For this review, take the finished solid that the model builds, in its own axes (mm). Face numbers are marked on the shaded views. A direction names the side the tool comes from. Round coordinates to 2 decimals unless told otherwise and drop trailing zeros. Write each loop counter-clockwise with the first axis right and the second up, starting at its lowest first coordinate (ties: lowest second). Pieces come first, ordered by that corner, then holes. Notation, with made-up numbers: (23, -32) -> (40, -32) arc R15 cw to (40, -13) -> close; hole circle Ø4 at (-10.5, -26). An arc over 180 degrees is marked (long way). Answer as CSV lines item,"result". Start each with the question number.
Item 1: Machinability: for the marked faces 5, 6, 7, 8 and 9, which of the approach directions +Z, -Z, +X, -X, +Y, -Y give a long, thin tool a straight path to every point of the face, cutting with its end or side? Answer none if there is none.
Item 2: For pin 1 Ø4 at (y, z) = (-1.5, -1.5) entering from +X; pin 2 Ø5 at (x, z) = (15, 1) entering from -Y; pin 3 Ø3 at (y, z) = (-8, -0.5) entering from -X, all flat-tipped, find the tip position at first contact; note any pin that passes through.
Item 3: Take a section at C-C on y = -9. Give the boundary of the cut face in (x, z).
Item 4: Take a section at D-D on x = 5. Give the boundary of the cut face in (y, z).
Item 5: Wall thickness on probe 1 along X at (y, z) = (-2.5, -2.25); probe 2 along X at (y, z) = (-2.5, -5.65); probe 3 along Z at (x, y) = (40, -11.5): over which ranges is each line inside the solid? List them lowest first. Write a range as from..to.
Item 6: Take a section at B-B on z = -0.5. Give the boundary of the cut face in (x, y).
Item 7: Mouldability with a two-part tool opening along Z and no side actions: class the marked faces 1, 2, 3 and 4 as +Z half, -Z half, draft (parallel to the pull), parting line (faces both ways), or undercut.
Item 8: Take a section at A-A on x = 34. Give the boundary of the cut face in (y, z), then the cut area to 3 significant figures.
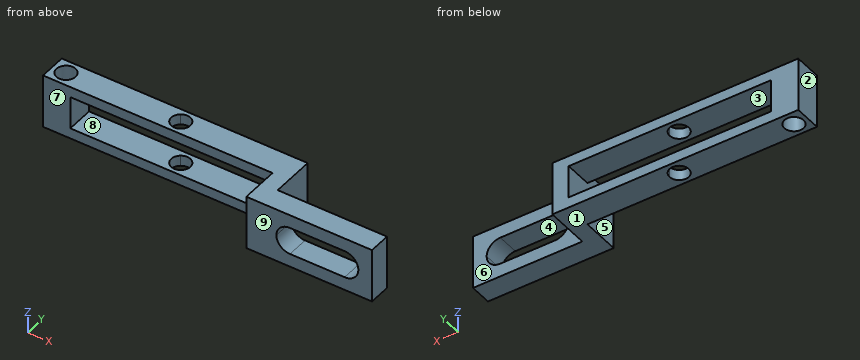
```python
from build123d import *

# Parameters (mm, degrees)
F0_W     = 3
F0_H     = 3
F1_DEPTH = 5
F3_DEPTH = 25
F4_W     = 3
F4_H     = 9.87
F5_DEPTH = 7
F6_W     = 4
F6_H     = 9.87
F7_DEPTH = 20
F9_DEPTH = 25


with BuildPart() as f1:
    # F0 (on Front) → F1 (new body)
    with BuildSketch(Plane.XZ):
        Polygon((-18.4640498906, -4.8765387449), (-18.4640498906, -6.8115387449), (26.5359501094, -6.8115387449), (26.5359501094, -4.8765387449), (23.5359501094, -4.8765387449), (-13.4640498906, -4.8765387449), align=None)
        Polygon((-18.4640498906, 3.0584612551), (-18.4640498906, -4.8765387449), (-13.4640498906, -4.8765387449), (-13.4640498906, 1.1234612551), (-1.7127114115, 1.1234612551), (23.5359501094, 1.1234612551), (26.5359501094, 1.1234612551), (26.5359501094, 3.0584612551), align=None)
        with Locations((25.0359501094, -3.3765387449)):
            Rectangle(F0_W, F0_H)
        with Locations((25.0359501094, -0.3765387449)):
            Rectangle(F0_W, F0_H)
    extrude(amount=F1_DEPTH)

    # F2 (on face) → F3 (cut)
    with BuildSketch(Plane.XY.offset(3.0584612551)):
        with BuildLine():
            ThreePointArc((-14.2140498906, -2.5), (-15.9640498906, -0.75), (-17.7140498906, -2.5))
            ThreePointArc((-17.7140498906, -2.5), (-15.9640498906, -4.25), (-14.2140498906, -2.5))
        make_face()
        with BuildLine():
            ThreePointArc((6.7859501094, -2.5), (5.8460426967, -0.9487907943), (4.0359501094, -1.0638593384))
            ThreePointArc((4.0359501094, -1.0638593384), (4.2258575221, -4.0512092057), (6.7859501094, -2.5))
        make_face()
    extrude(amount=-F3_DEPTH, mode=Mode.SUBTRACT)

    # F4 (on face) → F5 (join)
    with BuildSketch(Plane.XZ.offset(5)):
        with Locations((25.0359501094, -1.8765387449)):
            Rectangle(F4_W, F4_H)
    extrude(amount=F5_DEPTH)

    # F6 (on face) → F7 (join)
    with BuildSketch(Plane.YZ.offset(26.5359501094)):
        with Locations((-10, -1.8765387449)):
            Rectangle(F6_W, F6_H)
    extrude(amount=F7_DEPTH)

    # F8 (on face) → F9 (cut)
    with BuildSketch(Plane.XZ.offset(12)):
        with BuildLine():
            ThreePointArc((31.5359501094, 0.6234612551), (29.7681831564, -0.1087717919), (29.0359501094, -1.8765387449))
            Line((29.0359501094, -1.8765387449), (31.5359501094, -1.8765387449))
            Line((31.5359501094, -1.8765387449), (41.5359501094, -1.8765387449))
            Line((41.5359501094, -1.8765387449), (44.0359501094, -1.8765387449))
            ThreePointArc((44.0359501094, -1.8765387449), (43.3037170623, -0.1087717919), (41.5359501094, 0.6234612551))
            Line((41.5359501094, 0.6234612551), (31.5359501094, 0.6234612551))
        make_face()
        with BuildLine():
            Line((31.5359501094, -1.8765387449), (29.0359501094, -1.8765387449))
            ThreePointArc((29.0359501094, -1.8765387449), (29.7681831564, -3.6443056978), (31.5359501094, -4.3765387449))
            Line((31.5359501094, -4.3765387449), (41.5359501094, -4.3765387449))
            ThreePointArc((41.5359501094, -4.3765387449), (43.3037170623, -3.6443056978), (44.0359501094, -1.8765387449))
            Line((44.0359501094, -1.8765387449), (41.5359501094, -1.8765387449))
            Line((41.5359501094, -1.8765387449), (31.5359501094, -1.8765387449))
        make_face()
    extrude(amount=-F9_DEPTH, mode=Mode.SUBTRACT)


solid = f1.part
```
Output values:
1,face 5,"-Y"
1,face 6,"+Z, -Z, +X, +Y"
1,face 7,"+Z, -Z, -X, -Y"
1,face 8,"+Y, -Y"
1,face 9,"+Z, -Z, +X, -X, -Y"
2,pin 1,"stops at x = 26.54"
2,pin 2,"stops at y = -5"
2,pin 3,"stops at x = 23.54"
3,outline,"(23.54, -6.81) -> (46.54, -6.81) -> (46.54, 3.06) -> (23.54, 3.06) -> close; hole (31.54, -4.38) -> (41.54, -4.38) arc R2.5 ccw to (41.54, 0.62) -> (31.54, 0.62) arc R2.5 ccw to start"
4,outline,"(-5, -6.81) -> (-4.25, -6.81) -> (-4.25, -4.88) -> (-5, -4.88) -> close; (-5, 1.12) -> (-4.25, 1.12) -> (-4.25, 3.06) -> (-5, 3.06) -> close; (-0.75, -6.81) -> (0, -6.81) -> (0, -4.88) -> (-0.75, -4.88) -> close; (-0.75, 1.12) -> (0, 1.12) -> (0, 3.06) -> (-0.75, 3.06) -> close"
5,probe 1,"x = -18.46..-17.71, -14.21..-13.46, 23.54..26.54"
5,probe 2,"x = -18.46..-17.71, -14.21..3.29, 6.79..26.54"
5,probe 3,"z = -6.81..-4.38, 0.62..3.06"
6,outline,"(-18.46, -5) -> (-13.46, -5) -> (-13.46, 0) -> (-18.46, 0) -> close; (23.54, -12) -> (29.45, -12) -> (29.45, -8) -> (26.54, -8) -> (26.54, 0) -> (23.54, 0) -> close; (43.62, -12) -> (46.54, -12) -> (46.54, -8) -> (43.62, -8) -> close; hole circle Ø3.5 at (-15.96, -2.5)"
7,face 1,"-Z half"
7,face 2,"draft"
7,face 3,"undercut"
7,face 4,"undercut"
8,outline,"(-12, -6.81) -> (-8, -6.81) -> (-8, -4.38) -> (-12, -4.38) -> close; (-12, 0.62) -> (-8, 0.62) -> (-8, 3.06) -> (-12, 3.06) -> close"
8,area,"19.5 mm^2"
